```python
from build123d import *

# Parameters (mm, degrees)
SKETCH1_R           = 2.1
BOSS_EXTRUDE1_DEPTH = 1200


with BuildPart() as part:
    # Sketch1 → Boss-Extrude1 (new body)
    with BuildSketch(Plane(origin=(0, 0, -1000), x_dir=(-1, 0, 0), z_dir=(0, 0, -1))):
        with BuildLine():
            Line((10, -7), (10, 7))
            Line((10, 7), (8, 7))
            Line((8, 7), (8, 4))
            Line((8, 4), (7.060660172, 4))
            Line((7.060660172, 4), (4, 7.060660172))
            Line((4, 7.060660172), (4, 9.480384758))
            Line((4, 9.480384758), (3.7, 10))
            Line((3.7, 10), (4, 10.519615242))
            Line((4, 10.519615242), (4, 12.939339828))
            Line((4, 12.939339828), (7.060660172, 16))
            Line((7.060660172, 16), (8, 16))
            Line((8, 16), (8, 13))
            Line((8, 13), (10, 13))
            Line((10, 13), (10, 19))
            ThreePointArc((10, 19), (9.948683298, 19.316227766), (9.8, 19.6))
            Line((9.8, 19.6), (3, 19.6))
            Line((3, 19.6), (3, 18))
            Line((3, 18), (6, 18))
            Line((6, 18), (6, 17.060660172))
            Line((6, 17.060660172), (2.939339828, 14))
            Line((2.939339828, 14), (0.519615242, 14))
            Line((0.519615242, 14), (0, 13.7))
            Line((0, 13.7), (-0.519615242, 14))
            Line((-0.519615242, 14), (-2.939339828, 14))
            Line((-2.939339828, 14), (-6, 17.060660172))
            Line((-6, 17.060660172), (-6, 18))
            Line((-6, 18), (-3, 18))
            Line((-3, 18), (-3, 19.6))
            Line((-3, 19.6), (-9.8, 19.6))
            ThreePointArc((-9.8, 19.6), (-9.948683298, 19.316227766), (-10, 19))
            Line((-10, 19), (-10, 13))
            Line((-10, 13), (-8, 13))
            Line((-8, 13), (-8, 16))
            Line((-8, 16), (-7.060660172, 16))
            Line((-7.060660172, 16), (-4, 12.939339828))
            Line((-4, 12.939339828), (-4, 10.519615242))
            Line((-4, 10.519615242), (-3.7, 10))
            Line((-3.7, 10), (-4, 9.480384758))
            Line((-4, 9.480384758), (-4, 7.060660172))
            Line((-4, 7.060660172), (-7.060660172, 4))
            Line((-7.060660172, 4), (-8, 4))
            Line((-8, 4), (-8, 7))
            Line((-8, 7), (-10, 7))
            Line((-10, 7), (-10, -7))
            Line((-10, -7), (-8, -7))
            Line((-8, -7), (-8, -4))
            Line((-8, -4), (-7.060660172, -4))
            Line((-7.060660172, -4), (-4, -7.060660172))
            Line((-4, -7.060660172), (-4, -9.480384758))
            Line((-4, -9.480384758), (-3.7, -10))
            Line((-3.7, -10), (-4, -10.519615242))
            Line((-4, -10.519615242), (-4, -12.939339828))
            Line((-4, -12.939339828), (-7.060660172, -16))
            Line((-7.060660172, -16), (-8, -16))
            Line((-8, -16), (-8, -13))
            Line((-8, -13), (-10, -13))
            Line((-10, -13), (-10, -19))
            ThreePointArc((-10, -19), (-9.948683298, -19.316227766), (-9.8, -19.6))
            Line((-9.8, -19.6), (-3, -19.6))
            Line((-3, -19.6), (-3, -18))
            Line((-3, -18), (-6, -18))
            Line((-6, -18), (-6, -17.060660172))
            Line((-6, -17.060660172), (-2.939339828, -14))
            Line((-2.939339828, -14), (-0.519615242, -14))
            Line((-0.519615242, -14), (0, -13.7))
            Line((0, -13.7), (0.519615242, -14))
            Line((0.519615242, -14), (2.939339828, -14))
            Line((2.939339828, -14), (6, -17.060660172))
            Line((6, -17.060660172), (6, -18))
            Line((6, -18), (3, -18))
            Line((3, -18), (3, -19.6))
            Line((3, -19.6), (9.8, -19.6))
            ThreePointArc((9.8, -19.6), (9.948683298, -19.316227766), (10, -19))
            Line((10, -19), (10, -13))
            Line((10, -13), (8, -13))
            Line((8, -13), (8, -16))
            Line((8, -16), (7.060660172, -16))
            Line((7.060660172, -16), (4, -12.939339828))
            Line((4, -12.939339828), (4, -10.519615242))
            Line((4, -10.519615242), (3.7, -10))
            Line((3.7, -10), (4, -9.480384758))
            Line((4, -9.480384758), (4, -7.060660172))
            Line((4, -7.060660172), (7.060660172, -4))
            Line((7.060660172, -4), (8, -4))
            Line((8, -4), (8, -7))
            Line((8, -7), (10, -7))
        make_face()
        with Locations((0, -10)):
            Circle(SKETCH1_R, mode=Mode.SUBTRACT)
        with Locations((0, 10)):
            Circle(SKETCH1_R, mode=Mode.SUBTRACT)
        with BuildLine():
            Line((8, 1.7), (8, -1.7))
            ThreePointArc((8, -1.7), (7.912132034, -1.912132034), (7.7, -2))
            Line((7.7, -2), (7.063603897, -2))
            ThreePointArc((7.063603897, -2), (6.948798867, -2.02283614), (6.851471863, -2.087867966))
            Line((6.851471863, -2.087867966), (2.939339828, -6))
            Line((2.939339828, -6), (-2.939339828, -6))
            Line((-2.939339828, -6), (-6.851471863, -2.087867966))
            ThreePointArc((-6.851471863, -2.087867966), (-6.948798867, -2.02283614), (-7.063603897, -2))
            Line((-7.063603897, -2), (-7.7, -2))
            ThreePointArc((-7.7, -2), (-7.912132034, -1.912132034), (-8, -1.7))
            Line((-8, -1.7), (-8, 1.7))
            ThreePointArc((-8, 1.7), (-7.912132034, 1.912132034), (-7.7, 2))
            Line((-7.7, 2), (-7.063603897, 2))
            ThreePointArc((-7.063603897, 2), (-6.948798867, 2.02283614), (-6.851471863, 2.087867966))
            Line((-6.851471863, 2.087867966), (-2.939339828, 6))
            Line((-2.939339828, 6), (2.939339828, 6))
            Line((2.939339828, 6), (6.851471863, 2.087867966))
            ThreePointArc((6.851471863, 2.087867966), (6.948798867, 2.02283614), (7.063603897, 2))
            Line((7.063603897, 2), (7.7, 2))
            ThreePointArc((7.7, 2), (7.912132034, 1.912132034), (8, 1.7))
        make_face(mode=Mode.SUBTRACT)
    extrude(amount=-BOSS_EXTRUDE1_DEPTH)


solid = part.part
```
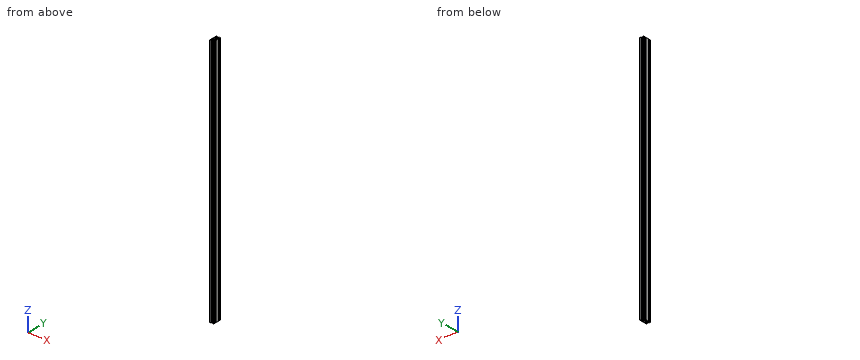
CAD build for the part. Positions are in the model's coordinates, mm. Round coordinates to 2 decimals unless told otherwise and drop trailing zeros.
Item 1: Band-saw the part on A-A on z = 81.5. Give the number of separate pieces and of enclosed holes in the cut face, then the cut area to 3 significant figures.
Filled in:
separate pieces: 1
enclosed holes: 3
area: 313 mm2
Item 2: Drill centre lines: L1, parallel to Y at x = 0, z = -400; L2, parallel to Y at x = 0.5, z = -765; L3, parallel to Y at x = 8.5, z = -199.5. Where is each one in solid material? Low to high.
Filled in:
L1: y = -13.7 to -12.1, -7.9 to -6, 6 to 7.9, 12.1 to 13.7
L2: y = -13.99 to -12.04, -7.96 to -6, 6 to 7.96, 12.04 to 13.99
L3: y = -19.6 to -13, -7 to 7, 13 to 19.6
Item 3: Drop flat-ended pins along their axis: pin 1 Ø2 at (x, y) = (5.5, -9.5) entering from -Z; pin 2 Ø0.7 at (y, z) = (8, -271.5) entering from +X. Give the stop position or say it passes through.
Filled in:
pin 1: passes through
pin 2: stops at x = 4
